from build123d import *

# Parameters (mm, degrees)
F1_DEPTH = 63.5
F0_W     = 25.4
F0_H     = 15.1617553278
F2_DEPTH = 25.4
F3_DEPTH = 7.9375
F5_R     = 6.35


with BuildPart() as f1:
    # F0 (on Front) → F1 (new body, symmetric)
    with BuildSketch(Plane.XZ):
        Polygon((-41.275, 9.525), (-41.275, -9.525), (41.275, -9.525), (41.275, 9.525), (22.225, 9.525), align=None)
    extrude(amount=F1_DEPTH, both=True)

    # F0 (on Front) → F2 (join, symmetric)
    with BuildSketch(Plane.XZ):
        with BuildLine():
            Line((22.225, 9.525), (41.275, 9.525))
            Line((41.275, 9.525), (41.275, 40.4134446722))
            ThreePointArc((41.275, 40.4134446722), (45.9246798487, 51.6387648236), (57.15, 56.2884446722))
            Line((57.15, 56.2884446722), (60.325, 56.2884446722))
            Line((60.325, 56.2884446722), (60.325, 71.4502))
            Line((60.325, 71.4502), (85.725, 71.4502))
            Line((85.725, 71.4502), (85.725, 75.3384446722))
            Line((85.725, 75.3384446722), (57.15, 75.3384446722))
            ThreePointArc((57.15, 75.3384446722), (32.4542956671, 65.1091490052), (22.225, 40.4134446722))
            Line((22.225, 40.4134446722), (22.225, 9.525))
        make_face()
        with Locations((73.025, 63.8693223361)):
            Rectangle(F0_W, F0_H)
    extrude(amount=F2_DEPTH, both=True)

    # F0 (on Front) → F3 (join, symmetric)
    with BuildSketch(Plane.XZ):
        with BuildLine():
            add(Edge.make_bspline(
                [(-41.275, 9.525), (-40.1609577239, 35.0168719888), (19.9037119746, 75.5567997694), (57.15, 75.3384446722)],
                knots=[0, 0, 0, 0, 118.4013940992, 118.4013940992, 118.4013940992, 118.4013940992], degree=3))
            Line((-41.275, 9.525), (22.225, 9.525))
            Line((22.225, 9.525), (22.225, 40.4134446722))
            ThreePointArc((22.225, 40.4134446722), (32.4542956671, 65.1091490052), (57.15, 75.3384446722))
        make_face()
    extrude(amount=F3_DEPTH, both=True)

    # F0 (on Front) → F4 (revolve)
    with BuildSketch(Plane.XZ):
        Polygon((111.125, 71.4502), (85.725, 71.4502), (85.725, 56.2884446722), (85.725, 42.8752), (111.125, 42.8752), align=None)
    revolve(axis=Axis((85.725, 0, 59.1068223361), (0, 0, 1)))

    # F5
    f5_edges = [f1.edges().sort_by_distance(p)[0] for p in [
        (41.275, -63.5, 0),
        (-41.275, -63.5, 0),
        (-41.275, 63.5, 0),
        (41.275, 63.5, 0),
    ]]
    fillet(f5_edges, radius=F5_R)


solid = f1.part
Can you work these out from the model? Positions are in its coordinate system, mm. A direction names the side the tool comes from. Round coordinates to 2 decimals unless told otherwise and drop trailing zeros. Loops run counter-clockwise (first coordinate to the right, second up) from the corner with the lowest first, then second, coordinate; pieces in that order, holes last. Notation, with made-up numbers: (-24, -13) - (-1, -13) arc R27 cw to (-1, 13) - close; hole circle Ø11 at (83, 7). An arc over 180 degrees is marked (long way). Write item = value, one per line. Start each with the question number.
(1) If I drill on probe 1 along Z at (x, y) = (69, -1); probe 2 along X at (y, z) = (-22, -1) (3 decimals); probe 3 along Z at (x, y) = (26.5, 26) (3 decimals), over which ranges is the centre line in solid material (lowest first)? Write a range as [from, to].
(2) For faces 1 (the face through (45.8, -0.36, 51.51)), 2 (the face through (41.275, -1, 10)), 3 (the face through (22.225, -17, 25)), 4 (the face through (60, 2, 56.288)), which set-ups out of +Z, -Z, +X, -X, +Y, -Y let a thin tool reach every point of the face, with its end or its side?
(3) If we section it at B-B (x = 101): Please give me the cut outline in (y, z), and give its area (3 significant figures).
(4) For P1, Ø2, axis at x = 78, y = 28, coming from the -Z side; P2, Ø20.5, axis at x = 103, y = 0, coming from the +Z side; P3, Ø4, axis at y = -19, z = 51.5, coming from the +X side; P4, Ø4, axis at x = -16.5, y = 45.5, coming from the +Z side (3 decimals), each with a flat end and sliding along its axis, tell me the tip position at first contact or that it passes through.
(5) If we section it at A-A (y = -54): Please give me the cut outline in (x, z) (3 decimals), and give its area (3 significant figures).
Ans:
q1.probe_1 = [42.88, 75.34]
q1.probe_2 = [-41.275, 41.275]
q1.probe_3 = [-9.525, 9.525]
q2.face_1 = -Z, +Y, -Y
q2.face_2 = -Z, +X, +Y, -Y
q2.face_3 = +Z, -X, -Y
q2.face_4 = -Z
q3.outline = (-20.29, 42.88) - (20.29, 42.88) - (20.29, 71.45) - (-20.29, 71.45) - close
q3.area = 1,160 mm²
q4.P1 = through
q4.P2 = 71.45
q4.P3 = 104.6
q4.P4 = 9.525
q5.outline = (-41.275, -9.525) - (41.275, -9.525) - (41.275, 9.525) - (-41.275, 9.525) - close
q5.area = 1,570 mm²
